Can you work these out from the model? Positions are in its coordinate system, mm. Face numbers are marked on the shaded views. A direction names the side the tool comes from. Round coordinates to 2 decimals unless told otherwise and drop trailing zeros. Order: outer loops, then holes, each group sorted by start corner. A loop starts at its lowest first (then second) coordinate and runs counter-clockwise, first axis right, second up. Notation, with made-up numbers: (-4, 59) -> (44, 59) arc R27 cw to (44, 93) -> close; hole circle Ø1 at (-15.75, 83.25). An arc over 180 degrees is marked (long way). One line per item, written item: value.
```python
from build123d import *

# Parameters (mm, degrees)
F0_W      = 129
F0_H      = 20
F1_DEPTH  = 12
F2_R      = 22.8473442097
F4_DEPTH  = 12
F3_R      = 35.3466345688
F5_DEPTH  = 12
F6_W      = 50.4865964812
F6_H      = 10
F7_DEPTH  = 12
F8_DEPTH  = 12
F9_R      = 4.99999
F11_DEPTH = 12
F13_DEPTH = 12
F14_R     = 5


# Not quite as in the source:
# - a fillet or chamfer is up to 0.001 mm smaller than in the source, because OpenCascade refuses the exact size


with BuildPart() as f1:
    # F0 (on Top) → F1 (new body)
    with BuildSketch(Plane.XY):
        with Locations((-0.2432982406, 9.9970398602)):
            Rectangle(F0_W, F0_H)
    extrude(amount=F1_DEPTH)

    # F2 (on Top) → F4 (join)
    with BuildSketch(Plane.XY):
        with Locations((-64.7432982406, 9.9970398602)):
            Circle(F2_R)
    extrude(amount=F4_DEPTH)

    # F3 (on Top) → F5 (join)
    with BuildSketch(Plane.XY):
        with Locations((64.2567017594, 9.9970398602)):
            Circle(F3_R)
    extrude(amount=F5_DEPTH)

    # F6 (on Top) → F7 (join)
    with BuildSketch(Plane.XY):
        with Locations((0, 10)):
            Rectangle(F6_W, F6_H)
    extrude(amount=F7_DEPTH)

    # F6 (on Top) → F8 (cut)
    with BuildSketch(Plane.XY):
        with Locations((0, 10)):
            Rectangle(F6_W, F6_H)
    extrude(amount=F8_DEPTH, mode=Mode.SUBTRACT)

    # F9 (radius 5 in the source; OpenCascade refuses exactly that, so slightly less here)
    f9_edges = [f1.edges().sort_by_distance(p)[0] for p in [
        (-25.243298, 15, 6),
        (25.243298, 15, 6),
        (25.243298, 5, 6),
        (-25.243298, 5, 6),
    ]]
    fillet(f9_edges, radius=F9_R)

    # F10 (on face) → F11 (cut)
    with BuildSketch(Plane.XY):
        Polygon((-60.7340801705, -3.0663675243), (-50.8161764394, 10.3375567669), (-60.499265179, 23.9120841357), (-76.4016468673, 18.8976791396), (-76.5467705132, 2.2240790499), align=None)
    extrude(amount=F11_DEPTH, mode=Mode.SUBTRACT)

    # F12 (on face) → F13 (cut)
    with BuildSketch(Plane.XY):
        Polygon((79.5819759369, -0.3051165918), (79.5819759369, 20.6023402938), (59.6978028267, 27.0630997807), (47.4087080063, 10.148611851), (59.6978028267, -6.7658760786), align=None)
    extrude(amount=F13_DEPTH, mode=Mode.SUBTRACT)

    # F14
    f14_edges = [f1.edges().sort_by_distance(p)[0] for p in [
        (-44.200632, -0.00296, 6),
        (30.354127, -0.00296, 6),
        (30.354127, 19.99704, 6),
        (-44.200632, 19.99704, 6),
    ]]
    fillet(f14_edges, radius=F14_R)


solid = f1.part
```
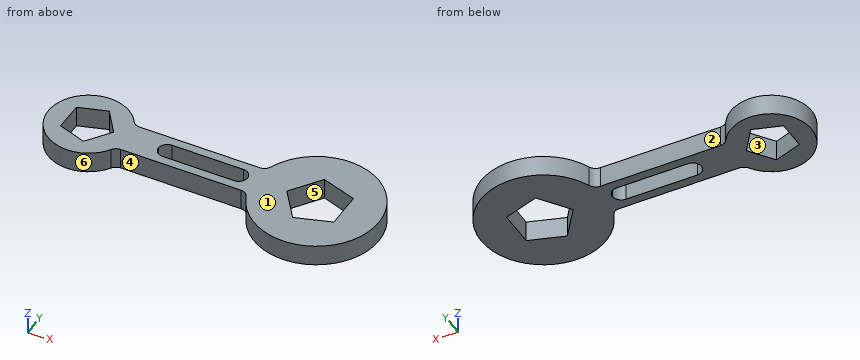
Q1. I want a section at A-A on x = 16.5. List the corners of the cut face in (y, z) for me, plus the area to 3 significant figures.
Answers below:
outline: (0, 0) -> (5, 0) -> (5, 12) -> (0, 12) -> close; (15, 0) -> (20, 0) -> (20, 12) -> (15, 12) -> close
area: 120 mm^2
Q2. We'd pull the mould along Y, two halves only. Please class the marked faces 4, 5 and 6: released by +Y, released by -Y, zero draft, split by the parting line, or undercut.
Answers below:
face 4: released by -Y
face 5: undercut
face 6: split by the parting line
Q3. On a 3-axis mill with a long thin cutter (end or side, diameter ignored), from which of +Z, -Z, +X, -X, +Y, -Y can I reach the whole of each face in a straight line? I mean the marked faces 1, 2 and 3. Say none if no direction works.
Answers below:
face 1: +Z, +X, -X, +Y, -Y
face 2: +Z, -Z, +Y
face 3: +Z, -Z
Q4. Will these pins go through, and if not, where does the flat tip stop? pin 1 Ø3 at (y, z) = (-9, 9.5) entering from -X; pin 2 Ø3.5 at (x, z) = (-9, 8) entering from -Y; pin 3 Ø6 at (y, z) = (28, 4) entering from -X.
Answers below:
pin 1: x = -79.44
pin 2: y = 0
pin 3: x = -81.97
Q5. Please list where these lines run through material, in increasing order: line 1 along Y through (x, z) = (4, 11); line 2 along Y through (x, z) = (-66, 2.75); line 3 along X through (y, z) = (-10, 8).
Answers below:
line 1: 0 to 5, 15 to 20
line 2: -12.82 to -1.3, 22.18 to 32.81
line 3: -75.79 to -53.69, 35.11 to 93.4
Q6. I want a section at C-C on z = 3. Give the number of separate pieces and of enclosed holes in the cut face, plus the area to 3 significant figures.
Answers below:
separate pieces: 1
enclosed holes: 3
area: 5,300 mm^2
Q7. I want a section at B-B on y = -10.5. List the corners of the cut face in (x, z) for me.
Answers below:
outline: (-74.84, 0) -> (-54.65, 0) -> (-54.65, 12) -> (-74.84, 12) -> close; (35.46, 0) -> (93.05, 0) -> (93.05, 12) -> (35.46, 12) -> close
